Check sheet for the modelled part. Datum: model origin and axes. Units: mm. Face numbers are marked on the shaded views. A direction names the side the tool comes from. Give positions to 0.01 mm unless a question says otherwise; leave off trailing zeros. Order: outer loops, then holes, each group sorted by start corner. A loop starts at its lowest first (then second) coordinate and runs counter-clockwise, first axis right, second up.
Autodesk Inventor part; units mm, degrees
ref_plane "YZ Plane" through (0, 0, 0) normal (1, 0, 0) x (0, 1, 0)
ref_plane "XZ Plane" through (0, 0, 0) normal (0, 1, 0) x (-1, 0, 0)
ref_plane "XY Plane" through (0, 0, 0) normal (0, 0, 1) x (1, 0, 0)
sketch "Sketch1" plane through (0, 0, 0) normal (0, 1, 0) x (-1, 0, 0)
  line L0 (63.5, 25.4) -> (-63.5, 25.4)
  line L1 (-63.5, 25.4) -> (-63.5, -25.4)
  line L2 (-63.5, -25.4) -> (63.5, -25.4)
  line L3 (63.5, -25.4) -> (63.5, 25.4)
  point P0 (0, 0)
  dimension "d0" = 50.8
  dimension "d1" = 25.4
  dimension "d2" = 63.5
  dimension "d3" = 127
extrude "Extrusion1" add sketch "Sketch1" along normal blind 6.35
sketch "Sketch2" plane through (0, 6.35, 0) normal (0, 1, 0) x (1, 0, 0)
  line L0 (-60.325, -22.225) -> (60.325, -22.225)
  line L1 (60.325, -22.225) -> (60.325, 22.225)
  line L2 (60.325, 22.225) -> (-60.325, 22.225)
  line L3 (-60.325, 22.225) -> (-60.325, -22.225)
  line L4 (-63.5, -25.4) -> (63.5, -25.4)
  line L5 (63.5, -25.4) -> (63.5, 25.4)
  line L6 (63.5, 25.4) -> (-63.5, 25.4)
  line L7 (-63.5, 25.4) -> (-63.5, -25.4)
  point P0 (0, 0)
  dimension "d6" = 3.175
  dimension "d7" = 3.175
  dimension "d8" = 3.175
  dimension "d9" = 3.175
extrude "Extrusion2" add sketch "Sketch2" along normal blind 38.1
fillet "Fillet1" radius 3.175 4 edges at (-60.325, 25.4, -22.225) (60.325, 25.4, -22.225) (60.325, 25.4, 22.225) (-60.325, 25.4, 22.225)
sketch "Sketch4" plane through (63.5, 0, -25.4) normal (0, 0, -1) x (-1, 0, 0)
  line L0 (127, 0) -> (127, 44.45)
  line L1 (127, 44.45) -> (104.775, 44.45)
  line L2 (104.775, 44.45) -> (104.775, 38.1)
  line L3 (104.775, 38.1) -> (127, 38.1)
  line L4 (127, 38.1) -> (127, 44.45)
  line L5 (74.6125, 44.45) -> (52.3875, 44.45)
  line L6 (52.3875, 44.45) -> (52.3875, 38.1)
  line L7 (52.3875, 38.1) -> (74.6125, 38.1)
  line L8 (74.6125, 38.1) -> (74.6125, 44.45)
  line L9 (22.225, 44.45) -> (0, 44.45)
  line L10 (0, 44.45) -> (0, 38.1)
  line L11 (0, 38.1) -> (22.225, 38.1)
  line L12 (22.225, 38.1) -> (22.225, 44.45)
  point P0 (63.5, 0)
  dimension "d28" = 22.225
  dimension "d29" = 6.35
  dimension "d32" = 52.3875
extrude "Extrusion4" [suppressed]
sketch "Sketch5" plane through (-63.5, 0, -25.4) normal (-1, 0, 0) x (0, 0, 1)
  line L0 (-15.24, 38.1) -> (0, 22.86)
  line L1 (0, 0) -> (0, 44.45)
  line L2 (0, 44.45) -> (0, 38.1)
  line L3 (0, 22.86) -> (0, 38.1)
  line L4 (0, 38.1) -> (-15.24, 38.1)
  point P0 (25.4, 0)
  dimension "d39" = 15.24
extrude "Extrusion5" [suppressed]
pattern_linear "Rectangular Pattern1" [suppressed]
pattern_linear "Rectangular Pattern2" [suppressed]
sketch "Sketch6" plane through (-60.325, 38.1, -40.64) normal (0, -1, 0) x (1, 0, 0)
  line L0 (123.825, 15.24) -> (-3.175, 15.24)
  line L1 (15.875, 0) -> (0, 0)
  line L2 (15.875, 0) -> (15.875, 15.24)
  line L3 (0, 15.24) -> (0, 0)
  point P0 (60.325, 40.64)
  point P1 (7.9375, 7.62)
  point P2 (60.3377, 7.62)
  point P3 (112.7379, 7.62)
  dimension "d48" = 7.62
  dimension "d49" = 15.24
  dimension "d50" = 15.875
  dimension "d51" = 7.9375
  dimension "d54" = 52.4002
hole "Hole1" [suppressed]
fillet "Fillet2" [suppressed]
fillet "Fillet3" [suppressed]
mirror "Mirror1" [suppressed]
fillet "Fillet4" [suppressed]
sketch "Sketch13" plane through (0, 44.45, 0) normal (0, 1, 0) x (1, 0, 0)
  line L0 (-74.295, 36.195) -> (74.295, 36.195)
  line L1 (74.295, 36.195) -> (74.295, -36.195)
  line L2 (74.295, -36.195) -> (-74.295, -36.195)
  line L3 (-74.295, -36.195) -> (-74.295, 36.195)
  line L4 (63.5, 25.4) -> (-63.5, 25.4)
  line L5 (-63.5, 25.4) -> (-63.5, -25.4)
  line L6 (-63.5, -25.4) -> (63.5, -25.4)
  line L7 (63.5, -25.4) -> (63.5, 25.4)
  point P0 (0, 0)
  dimension "d81" = 10.795
  dimension "d82" = 10.795
  dimension "d83" = 10.795
  dimension "d84" = 10.795
extrude "Extrusion12" add sketch "Sketch13" against normal blind 6.35
fillet "Fillet6" radius 3.175 4 edges at (-74.295, 41.275, -36.195) (74.295, 41.275, -36.195) (74.295, 41.275, 36.195) (-74.295, 41.275, 36.195)
sketch "Sketch14" plane through (0, 38.1, 0) normal (0, -1, 0) x (1, 0, 0)
  line L0 (74.295, 36.195) -> (-74.295, 36.195)
  line L1 (66.675, 28.575) -> (-66.675, 28.575)
  line L2 (74.295, -36.195) -> (74.295, 36.195)
  line L3 (74.295, -36.195) -> (74.295, 36.195)
  line L4 (74.295, 0) -> (-74.2494, 0) construction
  line L5 (71.12, -36.195) -> (-71.12, -36.195)
  line L6 (66.675, -28.575) -> (66.675, 28.575)
  line L7 (-74.295, -36.195) -> (74.295, -36.195)
  line L8 (0, -36.195) -> (0, 36.195) construction
  point P0 (0, 0)
  point P1 (59.2667, 32.385)
  point P2 (71.12, 36.195)
  point P3 (-71.12, 36.195)
  point P4 (74.295, -33.02)
  point P5 (74.295, 33.02)
  point P6 (44.45, 32.385)
  point P7 (29.6333, 32.385)
  point P8 (14.8167, 32.385)
  point P9 (0, 32.385)
  point P10 (-14.8167, 32.385)
  point P11 (-29.6333, 32.385)
  point P12 (-44.45, 32.385)
  point P13 (-59.2667, 32.385)
  point P14 (59.2667, -32.385)
  point P15 (44.45, -32.385)
  point P16 (29.6333, -32.385)
  point P17 (14.8167, -32.385)
  point P18 (0, -32.385)
  point P19 (-14.8167, -32.385)
  point P20 (-29.6333, -32.385)
  point P21 (-44.45, -32.385)
  point P22 (-59.2667, -32.385)
  point P23 (70.485, -28.956)
  point P24 (70.485, -14.478)
  point P25 (70.485, 0)
  point P26 (70.485, 14.478)
  point P27 (70.485, 28.956)
  point P28 (-70.485, -28.956)
  point P29 (-70.485, -14.478)
  point P30 (-70.485, 0)
  point P31 (-70.485, 14.478)
  point P32 (-70.485, 28.956)
  dimension "d88" = 3.81
  dimension "d89" = 7.62
  dimension "d94" = 14.8167
  dimension "d99" = 118.5333
  dimension "d100" = 59.2667
  dimension "d101" = 7.62
  dimension "d102" = 3.81
  dimension "d103" = 7.239
  dimension "d106" = 14.478
  dimension "d128" = 57.912
  dimension "d129" = 28.956
hole "Hole2" at (59.2667, 38.1, 32.385) at (44.45, 38.1, 32.385) at (29.6333, 38.1, 32.385) at (14.8167, 38.1, 32.385) at (0, 38.1, 32.385) at (-14.8167, 38.1, 32.385) at (-29.6333, 38.1, 32.385) at (-44.45, 38.1, 32.385) at (-59.2667, 38.1, 32.385) at (-59.2667, 38.1, -32.385) at (-44.45, 38.1, -32.385) at (-29.6333, 38.1, -32.385) at (-14.8167, 38.1, -32.385) at (0, 38.1, -32.385) at (14.8167, 38.1, -32.385) at (29.6333, 38.1, -32.385) at (44.45, 38.1, -32.385) at (59.2667, 38.1, -32.385) at (70.485, 38.1, -28.956) at (70.485, 38.1, -14.478) at (70.485, 38.1, 0) at (70.485, 38.1, 14.478) at (70.485, 38.1, 28.956) at (-70.485, 38.1, 28.956) at (-70.485, 38.1, 14.478) at (-70.485, 38.1, 0) at (-70.485, 38.1, -14.478) at (-70.485, 38.1, -28.956) direction (0, 1, 0) diameter 2.9464 depth 25.4 tip angle 118
sketch "Sketch17" plane through (0, 0, 0) normal (0, -1, 0) x (1, 0, 0)
  line L0 (50.4, -14.25) -> (43.6, -14.25)
  line L1 (43.6, -14.25) -> (43.6, 9.75)
  line L2 (43.6, 9.75) -> (50.4, 9.75)
  line L3 (50.4, 9.75) -> (50.4, -14.25)
  point P0 (0, 0)
extrude "Extrusion14" cut sketch "Sketch17" against normal blind 6.35
sketch "Sketch18" plane through (0, 0, 0) normal (0, -1, 0) x (1, 0, 0)
  line L0 (59.29, -7.85) -> (52.49, -7.85)
  line L1 (52.49, -7.85) -> (52.49, 5.95)
  line L2 (52.49, 5.95) -> (59.29, 5.95)
  line L3 (59.29, 5.95) -> (59.29, -7.85)
  line L4 (-56.75, -4.3) -> (-49.95, -4.3)
  line L5 (-49.95, -4.3) -> (-49.95, -14.2)
  line L6 (-49.95, -14.2) -> (-56.75, -14.2)
  line L7 (-56.75, -14.2) -> (-56.75, -4.3)
  point P0 (0, 0)
extrude "Extrusion15" cut sketch "Sketch18" against normal through all
sketch "Sketch19" plane through (0, 0, 0) normal (0, -1, 0) x (1, 0, 0)
  circle A0 centre (55.89, 8.15) radius 1.6
  circle A1 centre (55.89, -10.05) radius 1.6
  circle A2 centre (-53.35, -2.1) radius 1.6
  circle A3 centre (-53.35, -16.4) radius 1.6
  circle A4 centre (47, -16.4) radius 1.6
  circle A5 centre (47, 11.9) radius 1.6
  point P0 (0, 0)
extrude "Extrusion16" cut sketch "Sketch19" against normal through all
sketch "Sketch20" plane through (0, 44.45, 0) normal (0, 1, 0) x (1, 0, 0)
  circle A0 centre (47, 16.4) radius 1.6
  circle A1 centre (-53.35, 2.1) radius 1.6
  circle A2 centre (55.89, -8.15) radius 1.6
  circle A3 centre (55.89, 10.05) radius 1.6
  circle A4 centre (-53.35, 16.4) radius 1.6
  circle A5 centre (47, -11.9) radius 1.6
  line L0 (-56.75, 4.3) -> (-56.75, 14.2)
  line L1 (-56.75, 14.2) -> (-49.95, 14.2)
  line L2 (-49.95, 14.2) -> (-49.95, 4.3)
  line L3 (-49.95, 4.3) -> (-56.75, 4.3)
  line L4 (59.29, 7.85) -> (59.29, -5.95)
  line L5 (59.29, -5.95) -> (52.49, -5.95)
  line L6 (52.49, -5.95) -> (52.49, 7.85)
  line L7 (52.49, 7.85) -> (59.29, 7.85)
  line L8 (50.4, 14.25) -> (50.4, -9.75)
  line L9 (50.4, -9.75) -> (43.6, -9.75)
  line L10 (43.6, -9.75) -> (43.6, 14.25)
  line L11 (43.6, 14.25) -> (50.4, 14.25)
  arc A6 (-60.325, -19.05) -> (-57.15, -22.225) centre (-57.15, -19.05) ccw
  line L12 (-57.15, -22.225) -> (57.15, -22.225)
  arc A7 (57.15, -22.225) -> (60.325, -19.05) centre (57.15, -19.05) ccw
  line L13 (60.325, -19.05) -> (60.325, 19.05)
  arc A8 (60.325, 19.05) -> (57.15, 22.225) centre (57.15, 19.05) ccw
  line L14 (57.15, 22.225) -> (-57.15, 22.225)
  arc A9 (-57.15, 22.225) -> (-60.325, 19.05) centre (-57.15, 19.05) ccw
  line L15 (-60.325, 19.05) -> (-60.325, -19.05)
  line L16 (-57.15, 24.9809) -> (57.15, 24.9809)
  arc A10 (63.0809, 19.05) -> (57.15, 24.9809) centre (57.15, 19.05) ccw
  line L17 (63.0809, 19.05) -> (63.0809, -19.05)
  arc A11 (57.15, -24.9809) -> (63.0809, -19.05) centre (57.15, -19.05) ccw
  line L18 (57.15, -24.9809) -> (-57.15, -24.9809)
  arc A12 (-63.0809, -19.05) -> (-57.15, -24.9809) centre (-57.15, -19.05) ccw
  line L19 (-63.0809, -19.05) -> (-63.0809, 19.05)
  arc A13 (-57.15, 24.9809) -> (-63.0809, 19.05) centre (-57.15, 19.05) ccw
  line L20 (57.15, 28.1559) -> (-57.15, 28.1559)
  arc A14 (-57.15, 28.1559) -> (-66.2559, 19.05) centre (-57.15, 19.05) ccw
  line L21 (-66.2559, 19.05) -> (-66.2559, -19.05)
  arc A15 (-66.2559, -19.05) -> (-57.15, -28.1559) centre (-57.15, -19.05) ccw
  line L22 (-57.15, -28.1559) -> (57.15, -28.1559)
  arc A16 (57.15, -28.1559) -> (66.2559, -19.05) centre (57.15, -19.05) ccw
  line L23 (66.2559, -19.05) -> (66.2559, 19.05)
  arc A17 (66.2559, 19.05) -> (57.15, 28.1559) centre (57.15, 19.05) ccw
  point P0 (0, 0)
  dimension "d130" = 2.7559
  dimension "d131" = 3.175
extrude "Extrusion18" cut sketch "Sketch20" against normal blind 2.032 contours A17 L23 A16 L22 A15 L21 A14 L20
fillet "Fillet7" radius 3.175 4 edges at (-63.5, 19.05, -25.4) (63.5, 19.05, -25.4) (63.5, 19.05, 25.4) (-63.5, 19.05, 25.4)
equation "\"d7\" = d6"
equation "\"d8\" = d6"
equation "\"d9\" = d6"
equation "\"d81\" = d83"
equation "\"d82\" = d83"
equation "\"d84\" = d83"
properties part number "Electronics Box" material "Aluminum 6061"
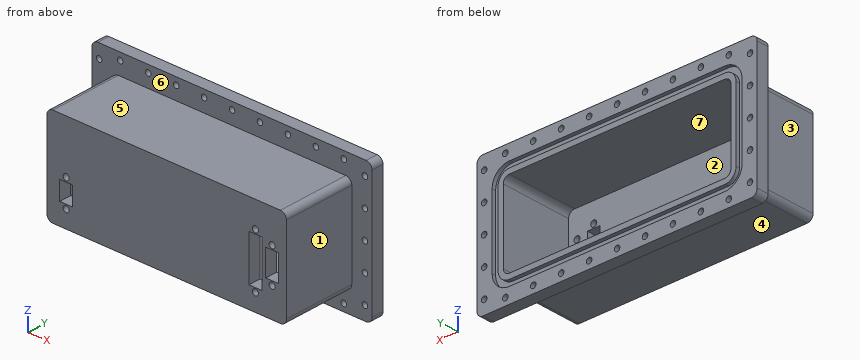
(1) Cross-section at B-B on x = -53.35. Count the separate pieces of the cut face and the enclosed holes in it, then the cut area to 3 significant figures.
Response values:
separate pieces: 4
enclosed holes: 0
area: 585 mm2
(2) Cross-section at A-A on z = 8.15. Enter the section's corners in (x, y) (3 decimals).
Response values:
outline: (-74.295, 38.1) - (-63.5, 38.1) - (-63.5, 0) - (43.6, 0) - (43.6, 6.35) - (-60.325, 6.35) - (-60.325, 44.45) - (-63.081, 44.45) - (-63.081, 42.418) - (-66.256, 42.418) - (-66.256, 44.45) - (-74.295, 44.45) - close; (50.4, 0) - (54.29, 0) - (54.29, 6.35) - (50.4, 6.35) - close; (57.49, 0) - (63.5, 0) - (63.5, 38.1) - (74.295, 38.1) - (74.295, 44.45) - (66.256, 44.45) - (66.256, 42.418) - (63.081, 42.418) - (63.081, 44.45) - (60.325, 44.45) - (60.325, 6.35) - (57.49, 6.35) - close
(3) Gauge pin test, flat ends, axial feed: pin 1 Ø19 at (x, y) = (5.5, 27.5) entering from +Z; pin 2 Ø17 at (x, z) = (22, 3) entering from +Y; pin 3 Ø19 at (x, y) = (-14, 22) entering from -Z. Record the tip position at first contact, or that the pin passes through.
Response values:
pin 1: stops at z = 25.4
pin 2: stops at y = 6.35
pin 3: stops at z = -25.4
(4) Cross-section at D-D on x = 0. Enter the section's corners in (y, z) (3 decimals), then the cut area to 3 significant figures.
Response values:
outline: (0, -25.4) - (38.1, -25.4) - (38.1, -30.912) - (44.45, -30.912) - (44.45, -28.156) - (42.418, -28.156) - (42.418, -24.981) - (44.45, -24.981) - (44.45, -22.225) - (6.35, -22.225) - (6.35, 22.225) - (44.45, 22.225) - (44.45, 24.981) - (42.418, 24.981) - (42.418, 28.156) - (44.45, 28.156) - (44.45, 30.912) - (38.1, 30.912) - (38.1, 25.4) - (0, 25.4) - close; (38.1, -36.195) - (44.45, -36.195) - (44.45, -33.858) - (38.1, -33.858) - close; (38.1, 33.858) - (44.45, 33.858) - (44.45, 36.195) - (38.1, 36.195) - close
area: 651 mm2
(5) Release check for a two-part mould opening along Z. For the marked faces 5, 6 and 7 record: released by +Z, released by -Z, zero draft, split by the parting line, or undercut.
Response values:
face 5: released by +Z
face 6: zero draft
face 7: undercut
(6) Material ranges on L1, parallel to Z at x = -46.5, y = 43 (3 decimals); L2, parallel to X at y = 32, z = -7 (3 decimals); L3, parallel to Z at x = 36, y = 39 (3 decimals), recorded low to high.
Response values:
L1: z = -36.195 to -28.156, -24.981 to -22.225, 22.225 to 24.981, 28.156 to 36.195
L2: x = -63.5 to -60.325, 60.325 to 63.5
L3: z = -36.195 to -22.225, 22.225 to 36.195
(7) Set-up check for the marked faces 1, 2, 3 and 4: record each of +Z, -Z, +X, -X, +Y, -Y from which the full face is reachable in a straight line by a thin tool's end or side.
Response values:
face 1: +Z, -Z, +X, -Y
face 2: +Y
face 3: +Z, -Z, -X, -Y
face 4: -Z, +X, -X, -Y
(8) Cross-section at C-C on y = 12. Enter the section's corners in (x, z) (3 decimals).
Response values:
outline: (-63.5, -22.225) arc R3.175 ccw to (-60.325, -25.4) - (60.325, -25.4) arc R3.175 ccw to (63.5, -22.225) - (63.5, 22.225) arc R3.175 ccw to (60.325, 25.4) - (-60.325, 25.4) arc R3.175 ccw to (-63.5, 22.225) - close; hole (-60.325, -19.05) arc R3.175 ccw to (-57.15, -22.225) - (57.15, -22.225) arc R3.175 ccw to (60.325, -19.05) - (60.325, 19.05) arc R3.175 ccw to (57.15, 22.225) - (-57.15, 22.225) arc R3.175 ccw to (-60.325, 19.05) - close
